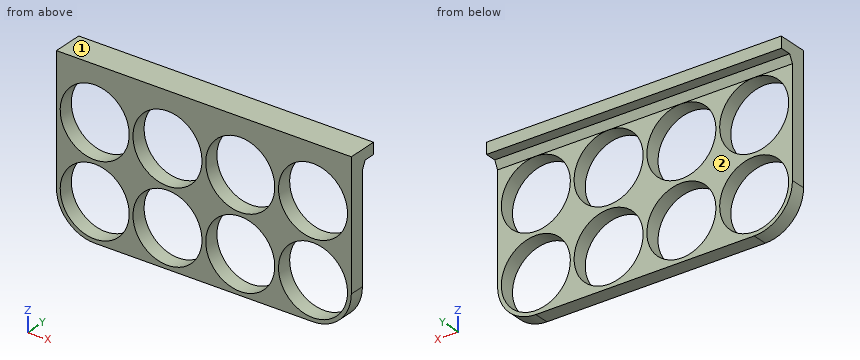
```python
from build123d import *

# Parameters (mm, degrees)
SKETCH1_R           = 9.2
BOSS_EXTRUDE1_DEPTH = 4
SKETCH2_W           = 78.6
SKETCH2_H           = 3
BOSS_EXTRUDE2_DEPTH = 4
BOSS_EXTRUDE3_DEPTH = 39.3


with BuildPart() as part:
    # Sketch1 → Boss-Extrude1 (new body)
    with BuildSketch(Plane(origin=(0, 0, 0), x_dir=(1, 0, 0), z_dir=(0, 1, 0))):
        with BuildLine():
            Line((-10.2, 0), (-10.2, -14.2))
            Line((-10.2, -14.2), (68.4, -14.2))
            Line((68.4, -14.2), (68.4, 0))
            Line((68.4, 0), (68.4, 19.4))
            ThreePointArc((68.4, 19.4), (65.412489168, 26.612489168), (58.2, 29.6))
            Line((58.2, 29.6), (0, 29.6))
            ThreePointArc((0, 29.6), (-7.212489168, 26.612489168), (-10.2, 19.4))
            Line((-10.2, 19.4), (-10.2, 0))
        make_face()
        with Locations(Location((0, 0, 0), (0, 0, 270))):
            Circle(SKETCH1_R, mode=Mode.SUBTRACT)
        with Locations(Location((19.4, 0, 0), (0, 0, 270))):
            Circle(SKETCH1_R, mode=Mode.SUBTRACT)
        with Locations(Location((38.8, 0, 0), (0, 0, 270))):
            Circle(SKETCH1_R, mode=Mode.SUBTRACT)
        with Locations(Location((58.2, 0, 0), (0, 0, 270))):
            Circle(SKETCH1_R, mode=Mode.SUBTRACT)
        with Locations(Location((19.4, 19.4, 0), (0, 0, 270))):
            Circle(SKETCH1_R, mode=Mode.SUBTRACT)
        with Locations(Location((38.8, 19.4, 0), (0, 0, 270))):
            Circle(SKETCH1_R, mode=Mode.SUBTRACT)
        with Locations(Location((58.2, 19.4, 0), (0, 0, 270))):
            Circle(SKETCH1_R, mode=Mode.SUBTRACT)
        with Locations(Location((0, 19.4, 0), (0, 0, 270))):
            Circle(SKETCH1_R, mode=Mode.SUBTRACT)
    extrude(amount=BOSS_EXTRUDE1_DEPTH)

    # Sketch2 → Boss-Extrude2 (add)
    with BuildSketch(Plane(origin=(0, 4, 0), x_dir=(1, 0, 0), z_dir=(0, 1, 0))):
        with Locations((29.1, -12.7)):
            Rectangle(SKETCH2_W, SKETCH2_H)
    extrude(amount=BOSS_EXTRUDE2_DEPTH)

    # Sketch3 → Boss-Extrude3 (add, symmetric)
    with BuildSketch(Plane(origin=(29.1, 0, 0), x_dir=(0, 0, -1), z_dir=(1, 0, 0))):
        Polygon((-9.2, 4), (-11.2, 5), (-11.2, 4), align=None)
    extrude(amount=BOSS_EXTRUDE3_DEPTH, both=True)


solid = part.part
```
For this review, take the finished solid that the model builds, in its own axes (mm). Face numbers are marked on the shaded views. A direction names the side the tool comes from. Round coordinates to 2 decimals unless told otherwise and drop trailing zeros. Order: outer loops, then holes, each group sorted by start corner. A loop starts at its lowest first (then second) coordinate and runs counter-clockwise, first axis right, second up.
Q1. Machinability: for the marked faces 1 and 2, which of the approach directions +Z, -Z, +X, -X, +Y, -Y give a long, thin tool a straight path to every point of the face, cutting with its end or side? Answer none if there is none.
Findings below:
face 1: +Z, +X, -X, +Y, -Y
face 2: -Z, +X, -X, +Y
Q2. We need section C-C, the plane z = 5. Give the boundary of the cut face in (x, y).
Findings below:
outline: (-10.2, 0) - (-7.72, 0) - (-7.72, 4) - (-10.2, 4) - close; (7.72, 0) - (11.68, 0) - (11.68, 4) - (7.72, 4) - close; (27.12, 0) - (31.08, 0) - (31.08, 4) - (27.12, 4) - close; (46.52, 0) - (50.48, 0) - (50.48, 4) - (46.52, 4) - close; (65.92, 0) - (68.4, 0) - (68.4, 4) - (65.92, 4) - close
Q3. Wall thickness on line 1 (Z direction, x = 39, y = 3.75); line 2 (X direction, y = 2.35, z = 0); line 3 (Z direction, x = 42, y = 3.25): over which ranges is each line inside the solid? List them lowest first.
Findings below:
line 1: z = -29.6 to -28.6, -10.2 to -9.2, 9.2 to 14.2
line 2: x = -10.2 to -9.2, 9.2 to 10.2, 28.6 to 29.6, 48 to 49, 67.4 to 68.4
line 3: z = -29.6 to -28.03, -10.77 to -8.63, 8.63 to 14.2
Q4. We need section D-D, the plane z = -7. Give the boundary of the cut face in (x, y).
Findings below:
outline: (-10.2, 0) - (-5.97, 0) - (-5.97, 4) - (-10.2, 4) - close; (5.97, 0) - (13.43, 0) - (13.43, 4) - (5.97, 4) - close; (25.37, 0) - (32.83, 0) - (32.83, 4) - (25.37, 4) - close; (44.77, 0) - (52.23, 0) - (52.23, 4) - (44.77, 4) - close; (64.17, 0) - (68.4, 0) - (68.4, 4) - (64.17, 4) - close
Q5. Insertion check: P1, Ø11, axis at x = 38.8, z = 0, coming from the -Y side; P2, Ø3.5, axis at x = 19.5, y = 7, coming from the -Z side; P3, Ø21, axis at x = 38.8, z = -19.4, coming from the +Y side. Each pin has a flat end and moves straight along its axis. Give the tip position at first contact, or say it passes through.
Findings below:
P1: passes through
P2: stops at z = 11.2
P3: stops at y = 4
Q6. We need section B-B, the plane x = -5. Give the boundary of the cut face in (y, z).
Findings below:
outline: (0, -28.29) - (4, -28.29) - (4, -27.12) - (0, -27.12) - close; (0, -11.68) - (4, -11.68) - (4, -7.72) - (0, -7.72) - close; (0, 7.72) - (4, 7.72) - (4, 9.2) - (5, 11.2) - (8, 11.2) - (8, 14.2) - (0, 14.2) - close
Q7. We need section A-A, the plane y = 1.5. State how many separate pieces and enclosed holes the cut face has, plus the area to 3 significant figures.
Findings below:
separate pieces: 1
enclosed holes: 8
area: 1,270 mm2
